Design review of the part built by this model. Coordinates are the model's own, in mm. A direction names the side the tool comes from. Coordinates: 2 decimals unless noted, no trailing zeros. Order: outer loops, then holes, each group sorted by start corner. A loop starts at its lowest first (then second) coordinate and runs counter-clockwise, first axis right, second up. Notation, with made-up numbers: M 74.5,35 L 122.5,35 A14 ccw 122.5,47 Z; hole C -7,86 d7. An arc over 180 degrees is marked long. Answer in a Markdown table with one row per item.
from build123d import *

# Parameters (mm, degrees)
F1_ANGLE = 200
F3_R     = 4
F3_R_2   = 8
F4_DEPTH = 15
F6_W     = 24
F6_H     = 6
F7_DEPTH = 25
F9_D     = 3
F9_DEPTH = 10


with BuildPart() as f1:
    # F0 (on Front) → F1 (revolve, symmetric)
    with BuildSketch(Plane.XZ) as f1_sk:
        Polygon((0, 7.5), (0, 5.5), (2, 5.5), (2, 11.5), (-26, 11.5), (-26, 5.5), (-24, 5.5), (-24, 7.5), align=None)
    revolve(axis=Axis((-13.749522, 0, 0), (1, 0, 0)), revolution_arc=F1_ANGLE / 2)
    revolve(f1_sk.sketch, axis=Axis((-13.749522, 0, 0), (-1, 0, 0)), revolution_arc=F1_ANGLE / 2)

    # F3 (on offset) → F4 (join)
    with BuildSketch(Plane.XY.offset(8)):
        with Locations((-12, 0)):
            Circle(F3_R)
        with Locations((-12, 0)):
            Circle(F3_R_2)
        with Locations((-12, 0)):
            Circle(F3_R, mode=Mode.SUBTRACT)
    extrude(amount=F4_DEPTH)

    # F6 (on offset) → F7 (join)
    with BuildSketch(Plane.XZ.offset(9)):
        with Locations((-12, 3)):
            Rectangle(F6_W, F6_H)
    extrude(amount=F7_DEPTH)

    # F9
    with Locations(Plane.XY.offset(6)):
        with Locations((-19, -29), (-5, -29), (-5, -17.000001), (-19, -17.000001)):
            Hole(F9_D / 2, depth=F9_DEPTH)


solid = f1.part
(1) Add section C-C, the plane x = -19. Give the boundary of the cut face in (y, z), and give its area (3 significant figures).
Return value:
| item | result |
|---|---|
| outline | M -34,0 L -30.5,0 L -30.5,6 L -34,6 Z; M -27.5,0 L -18.5,0 L -18.5,6 L -27.5,6 Z; M -15.5,0 L -11.5,0 A11.5 ccw -11.33,-2 L -7.39,-1.3 A7.5 cw long 7.39,-1.3 L 11.33,-2 A11.5 ccw 3.87,10.83 L 3.87,23 L -3.87,23 L -3.87,10.83 A11.5 ccw -9.81,6 L -15.5,6 Z |
| area | 326 mm2 |
(2) Add section D-D, the plane z = 12. Give the boundary of the cut face in (x, y).
Return value:
| item | result |
|---|---|
| outline | C -12,0 d16; hole C -12,0 d8 |
(3) Draft analysis for pull direction Y (two halves, no side actions). For faces 1 (the flat face through (-12, -34, 3)), 2 (the flat face through (-12, -22, 6)), 3 (the cylindrical face through (-20, 0, 17)), 4 (the flat face through (-24, 1, 6)), state which applies: pulls with the +Y half, pulls with the -Y half, needs draft (parallel to the pull), parting line crosses it, or undercut.
Return value:
| item | result |
|---|---|
| face 1 | pulls with the -Y half |
| face 2 | needs draft |
| face 3 | parting line crosses it |
| face 4 | undercut |
(4) Add section A-A, the plane y = -29. Give the boundary of the cut face in (x, z).
Return value:
| item | result |
|---|---|
| outline | M -24,0 L -20.5,0 L -20.5,6 L -24,6 Z; M -17.5,0 L -6.5,0 L -6.5,6 L -17.5,6 Z; M -3.5,0 L 0,0 L 0,6 L -3.5,6 Z |
(5) Add section B-B, the plane y = 0. Give the boundary of the cut face in (x, z).
Return value:
| item | result |
|---|---|
| outline | M -26,5.5 L -24,5.5 L -24,7.5 L 0,7.5 L 0,5.5 L 2,5.5 L 2,11.5 L -4,11.5 L -4,23 L -8,23 L -8,11.5 L -16,11.5 L -16,23 L -20,23 L -20,11.5 L -26,11.5 Z |
(6) Insertion check: pin 1 Ø6.5 at (y, z) = (0, 0) entering from -X; pin 2 Ø4.5 at (y, z) = (-3.5, 2) entering from -X; pin 3 Ø1.8 at (y, z) = (-26, 2) entering from -X; pin 4 Ø4 at (x, y) = (-19, -17) entering from +Z. Each pin has a flat end and moves straight along its axis. Give the tip position at first contact, or say it passes through.
Return value:
| item | result |
|---|---|
| pin 1 | passes through |
| pin 2 | stops at x = -26 |
| pin 3 | stops at x = -24 |
| pin 4 | stops at z = 6 |
(7) For faces 5 (the cylindrical face through (-11.832, -0.183, 7.498)), 6 (the flat face through (-12.2, -9.07, -1.6)), 7 (the flat face through (-12, -23, 0)), list the 3-axis set-ups (+Z, -Z, +X, -X, +Y, -Y) from which the entire face can be reached by the end or side of a thin tool; tool diameter is ignored.
Return value:
| item | result |
|---|---|
| face 5 | none |
| face 6 | -Z, +X, -X |
| face 7 | -Z, +X, -X, -Y |
(8) For line 1 along Y through (x, z) = (0.85, 0); line 2 along X through (y, z) = (-6, 4); line 3 along Z through (x, y) = (-10.75, -25), list the stretches that pass through material, from the lowest coordinate up. Write a range as from..to.
Return value:
| item | result |
|---|---|
| line 1 | y = -11.5..-5.5, 5.5..11.5 |
| line 2 | x = -26..-24, 0..2 |
| line 3 | z = 0..6 |
